from build123d import *

# Parameters (mm, degrees)
F0_W     = 150
F0_H     = 130
F1_DEPTH = 25
F2_T     = -2.5
F3_W     = 71.858019
F3_H     = 25
F4_DEPTH = 25


with BuildPart() as f1:
    # F0 (on Top) → F1 (new body)
    with BuildSketch(Plane.XY):
        Rectangle(F0_W, F0_H)
    extrude(amount=F1_DEPTH)

    # F2
    f2_openings = [f1.faces().sort_by_distance(p)[0] for p in [
        (0, 0, 25),
    ]]
    offset(amount=F2_T, openings=f2_openings)

    # F3 (on face) → F4 (cut)
    with BuildSketch(Plane.XZ.offset(65)):
        with Locations((-35.929009, 12.5)):
            Rectangle(F3_W, F3_H)
    extrude(amount=-F4_DEPTH, mode=Mode.SUBTRACT)


solid = f1.part
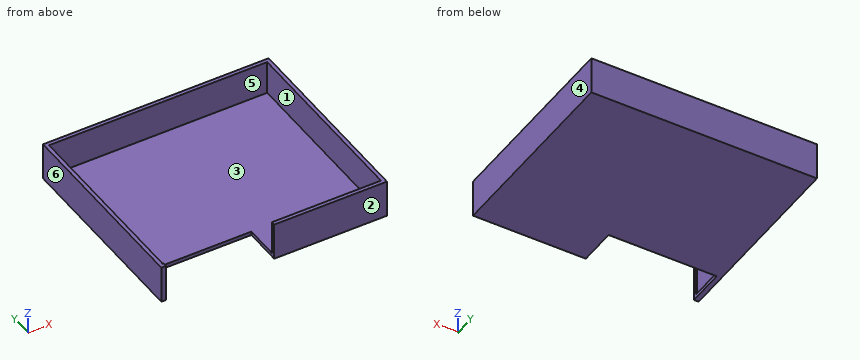
The listing builds one solid part. Answer for the finished solid, in the listing's coordinates (mm). Face numbers are marked on the shaded views. A direction names the side the tool comes from. Coordinates: 2 decimals unless noted, no trailing zeros. Write each loop counter-clockwise with the first axis right and the second up, starting at its lowest first coordinate (ties: lowest second). Pieces come first, ordered by that corner, then holes. Notation, with made-up numbers: M 88,-11.75 L 131,-11.75 A5 ccw 131,-3.75 Z; hole C -29.75,-13 d11. An arc over 180 degrees is marked long. Put each result on its own line as item: value. Start each with the question number.
1. A cutting plane is placed at B-B on z = 14. Write down the section's boundary in (x, y).
2. A cutting plane is placed at D-D on y = 20. Write down the section's boundary in (x, z).
3. Consider line 1 (X direction, y = -39.5, z = 21); line 2 (Y direction, x = 8.5, z = 15.5); line 3 (Z direction, x = -62, y = 19). Determine where each line is inside the solid, lowest interval first. Write a range as from..to.
4. A cutting plane is placed at C-C on x = 56. Write down the section's boundary in (y, z), then the cut area to 4 significant figures.
5. Which of the six approach directions +Z, -Z, +X, -X, +Y, -Y give full straight-line access (tool end or side, diameter ignored) to the marked faces 5 and 6?
6. For a pull along Y with two mould halves and no side action, classify the marked faces 1, 2, 3 and 4 as pulls with the +Y half, pulls with the -Y half, needs draft (parallel to the pull), parting line crosses it, or undercut.
7. Flat-ended cylindrical pins translate along their axes: P1, Ø1.5, axis at x = -0.5, y = -36, coming from the +Z side; P2, Ø3, axis at x = -35, z = 1.5, coming from the -Y side. Find the tip coordinate at first contact, or state that the pin passes through.
8. A cutting plane is placed at A-A on y = -47. Write down the section's boundary in (x, z).
Resolved:
1. outline: M -75,-65 L -71.86,-65 L -71.86,-62.5 L -72.5,-62.5 L -72.5,62.5 L 72.5,62.5 L 72.5,-62.5 L 0,-62.5 L 0,-65 L 75,-65 L 75,65 L -75,65 Z
2. outline: M -75,0 L 75,0 L 75,25 L 72.5,25 L 72.5,2.5 L -72.5,2.5 L -72.5,25 L -75,25 Z
3. line 1: x = -75..-72.5, 72.5..75
3. line 2: y = -65..-62.5, 62.5..65
3. line 3: z = 0..2.5
4. outline: M -65,0 L 65,0 L 65,25 L 62.5,25 L 62.5,2.5 L -62.5,2.5 L -62.5,25 L -65,25 Z
4. area: 437.5 mm2
5. face 5: +Z
5. face 6: +Z, -Z, -X, +Y, -Y
6. face 1: undercut
6. face 2: pulls with the -Y half
6. face 3: undercut
6. face 4: needs draft
7. P1: stops at z = 2.5
7. P2: stops at y = -40
8. outline: M -75,0 L -71.86,0 L -71.86,2.5 L -72.5,2.5 L -72.5,25 L -75,25 Z; M 0,0 L 75,0 L 75,25 L 72.5,25 L 72.5,2.5 L 0,2.5 Z
